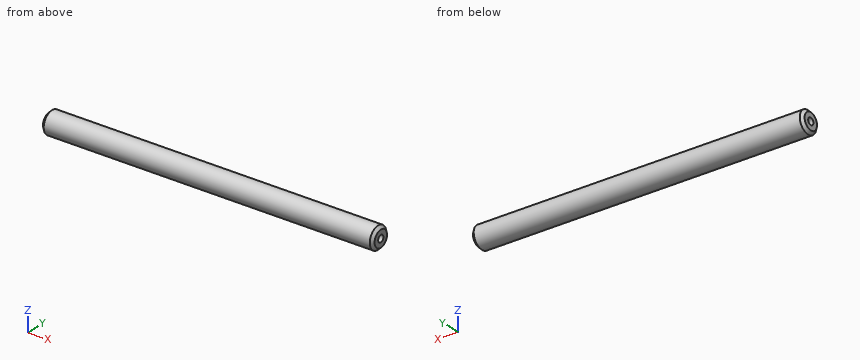
from build123d import *

# Parameters (mm, degrees)
ESQUISSE1_R           = 4
BOSS_EXTRU_1_DEPTH    = 60
CHANFREIN1_SIZE       = 1
TROU_TARAUD_M31_D     = 2.5
TROU_TARAUD_M31_DEPTH = 8.5
TROU_TARAUD_M31_TIP   = 0.751075774
TROU_TARAUD_M32_D     = 2.5
TROU_TARAUD_M32_DEPTH = 8.5
TROU_TARAUD_M32_TIP   = 0.751075774


with BuildPart() as part:
    # Esquisse1 → Boss.-Extru.1 (new, symmetric)
    with BuildSketch(Plane(origin=(0, 0, 0), x_dir=(0, 0, -1), z_dir=(1, 0, 0))):
        Circle(ESQUISSE1_R)
    extrude(amount=BOSS_EXTRU_1_DEPTH, both=True)

    # Chanfrein1
    chanfrein1_edges = [part.edges().sort_by_distance(p)[0] for p in [
        (-60, 0, 4),
        (60, 0, 4),
    ]]
    chamfer(chanfrein1_edges, length=CHANFREIN1_SIZE)

    # Trou taraudé M31
    with Locations(Plane(origin=(60, 0, 0), x_dir=(0, 0, -1), z_dir=(1, 0, 0))):
        with Locations((0, 0)):
            Hole(TROU_TARAUD_M31_D / 2, depth=TROU_TARAUD_M31_DEPTH)
            with Locations((0, 0, -(TROU_TARAUD_M31_DEPTH + TROU_TARAUD_M31_TIP / 2))):  # 118° drill point
                Cone(0, TROU_TARAUD_M31_D / 2, TROU_TARAUD_M31_TIP, mode=Mode.SUBTRACT)

    # Trou taraudé M32
    with Locations(Plane.ZY.offset(60)):
        with Locations((0, 0)):
            Hole(TROU_TARAUD_M32_D / 2, depth=TROU_TARAUD_M32_DEPTH)
            with Locations((0, 0, -(TROU_TARAUD_M32_DEPTH + TROU_TARAUD_M32_TIP / 2))):  # 118° drill point
                Cone(0, TROU_TARAUD_M32_D / 2, TROU_TARAUD_M32_TIP, mode=Mode.SUBTRACT)


solid = part.part
Input: part model. Units: mm. Frame: model coordinates. Give positions to 0.01 mm unless a question says otherwise; leave off trailing zeros. Loops run counter-clockwise (first coordinate to the right, second up) from the corner with the lowest first, then second, coordinate; pieces in that order, holes last. Notation, with made-up numbers: (77.25, -37) -> (136.25, -37) arc R8 ccw to (136.25, -22) -> close; hole circle Ø3 at (85, -36). An arc over 180 degrees is marked (long way). Answer as a JSON object with one key per item and string values. Group by question number.
Item 1: Line query: probe 1 along Y at (x, z) = (56, 0); probe 2 along Z at (x, y) = (-15, 0.25); probe 3 along Z at (x, y) = (34.5, -3.5). Output: solid intervals per line, ascending.
Item 2: Cut plane A-A, the plane x = -14. Return the cut outline in (y, z), and give its area (3 significant figures).
Item 3: Pin query (flat end, axial travel): P1, Ø2, axis at x = 42, z = 2.5, coming from the +Y side; P2, Ø3, axis at x = 32, y = 2.5, coming from the -Z side; P3, Ø1.5, axis at y = 0, z = 0, coming from the -X side. Return the tip coordinate at first contact, or that it passes through.
Checks:
{
 "1": {"probe 1": "y = -4 to -1.25, 1.25 to 4", "probe 2": "z = -3.99 to 3.99", "probe 3": "z = -1.94 to 1.94"},
 "2": {"outline": "circle Ø8 at (0, 0)", "area": "50.3 mm²"},
 "3": {"P1": "stops at y = 3.71", "P2": "stops at z = -3.87", "P3": "stops at x = -51.2"}
}
